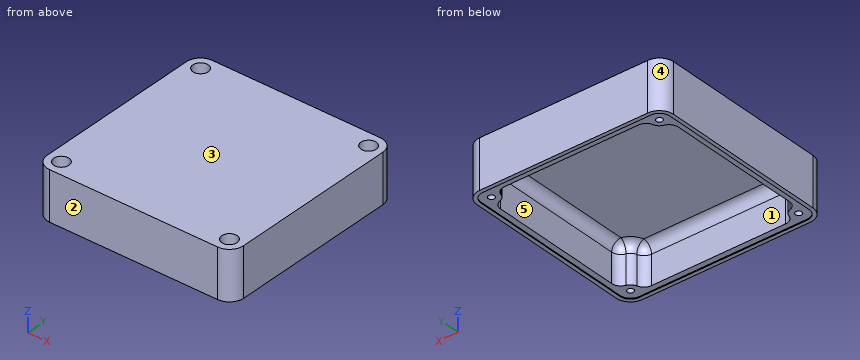
Autodesk Inventor part; units mm, degrees
ref_plane "YZ Plane" through (0, 0, 0) normal (1, 0, 0) x (0, 1, 0)
ref_plane "XZ Plane" through (0, 0, 0) normal (0, 1, 0) x (-1, 0, 0)
ref_plane "XY Plane" through (0, 0, 0) normal (0, 0, 1) x (1, 0, 0)
sketch "Skizze1" plane through (0, 0, 0) normal (0, 0, 1) x (1, 0, 0)
  line L0 (45, 50) -> (-45, 50)
  line L1 (-50, 45) -> (-50, -45)
  line L2 (-45, -50) -> (45, -50)
  line L3 (50, -45) -> (50, 45)
  line L4 (50, 50) -> (-50, -50) construction
  line L5 (-50, 50) -> (50, -50) construction
  arc A0 (45, -50) -> (50, -45) centre (45, -45) ccw
  arc A1 (-50, -45) -> (-45, -50) centre (-45, -45) ccw
  arc A2 (-45, 50) -> (-50, 45) centre (-45, 45) ccw
  arc A3 (50, 45) -> (45, 50) centre (45, 45) ccw
  line L6 (45, -50.6) -> (-45, -50.6)
  arc A4 (-50.6, -45) -> (-45, -50.6) centre (-45, -45) ccw
  line L7 (-50.6, -45) -> (-50.6, 45)
  arc A5 (-45, 50.6) -> (-50.6, 45) centre (-45, 45) ccw
  line L8 (-45, 50.6) -> (45, 50.6)
  arc A6 (50.6, 45) -> (45, 50.6) centre (45, 45) ccw
  line L9 (50.6, 45) -> (50.6, -45)
  arc A7 (45, -50.6) -> (50.6, -45) centre (45, -45) ccw
  line L10 (-45, -52.6) -> (45, -52.6)
  arc A8 (45, -52.6) -> (52.6, -45) centre (45, -45) ccw
  line L11 (52.6, -45) -> (52.6, 45)
  arc A9 (52.6, 45) -> (45, 52.6) centre (45, 45) ccw
  line L12 (45, 52.6) -> (-45, 52.6)
  arc A10 (-45, 52.6) -> (-52.6, 45) centre (-45, 45) ccw
  line L13 (-52.6, 45) -> (-52.6, -45)
  arc A11 (-52.6, -45) -> (-45, -52.6) centre (-45, -45) ccw
  point P0 (0, 0)
  point P1 (0, 0)
  dimension "d0" = 100
  dimension "d1" = 100
  dimension "d2" = 5
  dimension "d3" = 0.6
  dimension "d4" = 2
extrude "Extrusion1" add sketch "Skizze1" against normal blind 0.5 contours A11 L13 A10 L12 A9 L11 A8 L10
sketch "Skizze2" plane through (0, 0, 0) normal (0, 0, 1) x (1, 0, 0)
  line L0 (45, 52.6) -> (-45, 52.6)
  arc A0 (52.6, 45) -> (45, 52.6) centre (45, 45) ccw
  line L1 (52.6, -45) -> (52.6, 45)
  arc A1 (45, -52.6) -> (52.6, -45) centre (45, -45) ccw
  line L2 (-45, -52.6) -> (45, -52.6)
  arc A2 (-52.6, -45) -> (-45, -52.6) centre (-45, -45) ccw
  line L3 (-52.6, 45) -> (-52.6, -45)
  arc A3 (-45, 52.6) -> (-52.6, 45) centre (-45, 45) ccw
  line L4 (-41.4504, 47.6) -> (0, 47.6)
  line L5 (-47.6, 0) -> (-47.6, 41.4504)
  circle A4 centre (-45, 45) radius 1.7
  line L6 (-45, 50.6) -> (45, 50.6)
  line L7 (-50.6, -45) -> (-50.6, 45)
  arc A5 (-47.6, 41.4504) -> (-41.4504, 47.6) centre (-45, 45) ccw
  line L8 (-45, 52.6) -> (45, 52.6) construction
  line L9 (0, 52.6) -> (0, -52.6) construction
  line L10 (45, -52.6) -> (-45, -52.6) construction
  line L11 (-52.6, 0) -> (52.6, 0) construction
  line L12 (41.4504, 47.6) -> (0, 47.6)
  line L13 (47.6, 0) -> (47.6, 41.4504)
  circle A6 centre (45, 45) radius 1.7
  arc A7 (41.4504, 47.6) -> (47.6, 41.4504) centre (45, 45) ccw
  line L14 (-41.4504, -47.6) -> (0, -47.6)
  line L15 (-47.6, 0) -> (-47.6, -41.4504)
  circle A8 centre (-45, -45) radius 1.7
  arc A9 (-41.4504, -47.6) -> (-47.6, -41.4504) centre (-45, -45) ccw
  line L16 (47.6, 0) -> (47.6, -41.4504)
  arc A10 (47.6, -41.4504) -> (41.4504, -47.6) centre (45, -45) ccw
  circle A11 centre (45, -45) radius 1.7
  line L17 (41.4504, -47.6) -> (0, -47.6)
  point P0 (0, 0)
  dimension "d11" = 5
  dimension "d13" = 5
  dimension "d15" = 3.4
  dimension "d16" = 5.6
  dimension "d17" = 5.6
  dimension "d18" = 4.4
extrude "Extrusion2" add sketch "Skizze2" along normal blind 20.6
sketch "Skizze3" plane through (0, 0, 20.6) normal (0, 0, 1) x (1, 0, 0)
  line L0 (-52.6, 45) -> (-52.6, -45)
  arc A0 (-52.6, -45) -> (-45, -52.6) centre (-45, -45) ccw
  line L1 (-45, -52.6) -> (45, -52.6)
  arc A1 (45, -52.6) -> (52.6, -45) centre (45, -45) ccw
  line L2 (52.6, -45) -> (52.6, 45)
  arc A2 (52.6, 45) -> (45, 52.6) centre (45, 45) ccw
  line L3 (45, 52.6) -> (-45, 52.6)
  arc A3 (-45, 52.6) -> (-52.6, 45) centre (-45, 45) ccw
  point P0 (0, 0)
extrude "Extrusion3" add sketch "Skizze3" along normal blind 5
fillet "Rundung1" radius 5 8 edges at (-47.6, 41.4504, 10.3) (-41.4504, 47.6, 10.3) (47.6, 41.4504, 10.3) (41.4504, 47.6, 10.3) (41.4504, -47.6, 10.3) (47.6, -41.4504, 10.3) (-41.4504, -47.6, 10.3) (-47.6, -41.4504, 10.3)
fillet "Rundung2" radius 5 16 edges at (-46.5612, 38.9625, 20.6) (-41.8887, 41.8887, 20.6) (-38.9625, 46.5612, 20.6) (0, 47.6, 20.6) (38.9625, 46.5612, 20.6) (41.8887, 41.8887, 20.6) (46.5612, 38.9625, 20.6) (47.6, 0, 20.6) (46.5612, -38.9625, 20.6) (41.8887, -41.8887, 20.6) (38.9625, -46.5612, 20.6) (0, -47.6, 20.6) (-38.9625, -46.5612, 20.6) (-41.8887, -41.8887, 20.6) (-46.5612, -38.9625, 20.6) (-47.6, 0, 20.6)
sketch "Skizze4" plane through (0, 0, 25.6) normal (0, 0, 1) x (1, 0, 0)
  arc A0 (-45, 52.6) -> (-52.6, 45) centre (-45, 45) ccw
  arc A1 (52.6, 45) -> (45, 52.6) centre (45, 45) ccw
  arc A2 (45, -52.6) -> (52.6, -45) centre (45, -45) ccw
  arc A3 (-52.6, -45) -> (-45, -52.6) centre (-45, -45) ccw
  circle A4 centre (-45, 45) radius 1.7
  circle A5 centre (-45, 45) radius 4.1
  circle A6 centre (45, 45) radius 4.1
  circle A7 centre (45, -45) radius 1.7
  circle A8 centre (45, -45) radius 4.1
  circle A9 centre (-45, -45) radius 1.7
  circle A10 centre (-45, -45) radius 4.1
  point P0 (0, 0)
  dimension "d25" = 8.2
  dimension "d26" = 8.2
  dimension "d27" = 8.2
  dimension "d28" = 8.2
extrude "ExtrusionSchraubenKopf" cut sketch "Skizze4" against normal blind 7.6 contours A4 | A5 | A6 | A7 | A8 | A9 | A10
sketch "Skizze5" plane through (0, 0, 0) normal (0, 0, -1) x (-1, 0, 0)
  circle A0 centre (45, 45) radius 1.7
  circle A1 centre (45, -45) radius 1.7
  circle A2 centre (-45, -45) radius 1.7
  circle A3 centre (-45, 45) radius 1.7
  point P0 (0, 0)
extrude "ExtrusionSchraubenLoch" cut sketch "Skizze5" against normal up to surface (25.6 mm away)
equation "\"d0\" = BP"
equation "\"d1\" = LP"
equation "\"d2\" = REP"
equation "\"d3\" = TM"
equation "\"d9\" = -0.5 * TM + 0.5 * HPt"
equation "\"d11\" = DW"
equation "\"d13\" = DW"
equation "\"d15\" = DL"
equation "\"d16\" = REP + TM"
equation "\"d17\" = REP + TM"
equation "\"d19\" = HPb + TM"
equation "\"d21\" = DW"
equation "\"d23\" = RR"
equation "\"d24\" = RR"
equation "\"d25\" = SKD + 2 * TM"
equation "\"d26\" = SKD + 2 * TM"
equation "\"d27\" = SKD + 2 * TM"
equation "\"d28\" = SKD + 2 * TM"
equation "\"d29\" = SKH + TM"
equation "\"BP\" = 100"
equation "\"LP\" = 100"
equation "\"REP\" = 5"
equation "\"TM\" = 0.6"
equation "\"DW\" = 5"
equation "\"DL\" = 3.4"
equation "\"HPt\" = 1.6"
equation "\"HPb\" = 20"
equation "\"RR\" = 5"
equation "\"SKD\" = 7"
equation "\"SKH\" = 7"
properties part number "GehauseGenerator_GehauseVorlage"
Build history of the part. All positions in model axes, mm. Face numbers are marked on the shaded views. A direction names the side the tool comes from. Round coordinates to 2 decimals unless told otherwise and drop trailing zeros. Order: outer loops, then holes, each group sorted by start corner. A loop starts at its lowest first (then second) coordinate and runs counter-clockwise, first axis right, second up. Notation, with made-up numbers: (14, 35.25) - (56, 35.25) arc R24 cw to (56, 71.25) - close; hole circle Ø1 at (27, 23.25). An arc over 180 degrees is marked (long way). Use a Markdown table: item, result.
1) Saw through at A-A on z = 7.5. Write the cut outline in (x, y), and give its area (3 significant figures).
Recorded:
| item | result |
|---|---|
| outline | (-52.6, -45) arc R7.6 ccw to (-45, -52.6) - (45, -52.6) arc R7.6 ccw to (52.6, -45) - (52.6, 45) arc R7.6 ccw to (45, 52.6) - (-45, 52.6) arc R7.6 ccw to (-52.6, 45) - close; hole (-47.6, -35.91) arc R5 ccw to (-43.88, -40.75) arc R4.4 cw to (-40.75, -43.88) arc R5 ccw to (-35.91, -47.6) - (35.91, -47.6) arc R5 ccw to (40.75, -43.88) arc R4.4 cw to (43.88, -40.75) arc R5 ccw to (47.6, -35.91) - (47.6, 35.91) arc R5 ccw to (43.88, 40.75) arc R4.4 cw to (40.75, 43.88) arc R5 ccw to (35.91, 47.6) - (-35.91, 47.6) arc R5 ccw to (-40.75, 43.88) arc R4.4 cw to (-43.88, 40.75) arc R5 ccw to (-47.6, 35.91) - close; hole circle Ø3.4 at (-45, -45); hole circle Ø3.4 at (-45, 45); hole circle Ø3.4 at (45, -45); hole circle Ø3.4 at (45, 45) |
| area | 2,130 mm² |
2) Wall check: L1, parallel to Y at x = 18.5, z = 1.5; L2, parallel to X at y = -44, z = 1.5. Give the ranges that are in metal, low to high.
Recorded:
| item | result |
|---|---|
| L1 | y = -52.6 to -47.6, 47.6 to 52.6 |
| L2 | x = -52.6 to -46.37, -43.63 to -40.71, 40.71 to 43.63, 46.37 to 52.6 |
3) Saw through at B-B on y = 19. Write the cut outline in (x, z).
Recorded:
| item | result |
|---|---|
| outline | (-52.6, -0.5) - (-50.6, -0.5) - (-50.6, 0) - (-47.6, 0) - (-47.6, 15.6) arc R5 cw to (-42.6, 20.6) - (42.6, 20.6) arc R5 cw to (47.6, 15.6) - (47.6, 0) - (50.6, 0) - (50.6, -0.5) - (52.6, -0.5) - (52.6, 25.6) - (-52.6, 25.6) - close |
4) Pull direction X, two halves, no side cores. Call the marked faces 3, 4 and 5: pulls with the +X half, pulls with the -X half, needs draft (parallel to the pull), parting line crosses it, or undercut.
Recorded:
| item | result |
|---|---|
| face 3 | needs draft |
| face 4 | pulls with the -X half |
| face 5 | undercut |
5) Tool access for the marked faces 1 and 2: list every direction of +Z, -Z, +X, -X, +Y, -Y with a clear straight run to the whole face (end or side of a thin tool).
Recorded:
| item | result |
|---|---|
| face 1 | -Z |
| face 2 | +Z, -Z, +X, -X, -Y |
6) Flat gauge pins, fed straight in: pin 1 Ø5 at (x, y) = (45, 45) entering from +Z; pin 2 Ø2 at (x, y) = (-45, -45) entering from +Z; pin 3 Ø9.5 at (x, y) = (-45, 45) entering from -Z. Where does each tip first touch, or does it go through?
Recorded:
| item | result |
|---|---|
| pin 1 | stops at z = 18 |
| pin 2 | passes through |
| pin 3 | stops at z = 0 |
